Model file for the job. Use its own axes, mm. Face numbers are marked on the shaded views. A direction names the side the tool comes from. Coordinates: 2 decimals unless noted, no trailing zeros. Order: outer loops, then holes, each group sorted by start corner. A loop starts at its lowest first (then second) coordinate and runs counter-clockwise, first axis right, second up.
from build123d import *

# Parameters (mm, degrees)
MODEL_R                 = 1.5
MODEL_W                 = 3
MODEL_H                 = 3
SALIENTE_EXTRUIR1_DEPTH = 3


with BuildPart() as part:
    # Model → Saliente-Extruir1 (new body)
    with BuildSketch(Plane.XY):
        with BuildLine():
            Line((10.993657745, 286.638352596), (10.993657745, 280.893789949))
            ThreePointArc((10.993657745, 280.893789949), (11.107252484, 280.430879899), (11.422229173, 280.073138143))
            ThreePointArc((11.422229173, 280.073138143), (12.115845844, 279.676594232), (12.868657745, 279.408965008))
            ThreePointArc((12.868657745, 279.408965008), (14.499333705, 278.609421111), (15.681157745, 277.230411876))
            ThreePointArc((15.681157745, 277.230411876), (27.493657745, 270.266071273), (39.306157745, 277.230411876))
            ThreePointArc((39.306157745, 277.230411876), (40.487981784, 278.609421111), (42.118657745, 279.408965008))
            ThreePointArc((42.118657745, 279.408965008), (42.871469645, 279.676594232), (43.565086316, 280.073138143))
            ThreePointArc((43.565086316, 280.073138143), (43.880063005, 280.430879899), (43.993657745, 280.893789949))
            Line((43.993657745, 280.893789949), (43.993657745, 286.638352596))
            ThreePointArc((43.993657745, 286.638352596), (43.880063005, 287.101262646), (43.565086316, 287.459004403))
            ThreePointArc((43.565086316, 287.459004403), (42.871469645, 287.855548313), (42.118657745, 288.123177537))
            ThreePointArc((42.118657745, 288.123177537), (40.487981784, 288.922721434), (39.306157745, 290.301730669))
            ThreePointArc((39.306157745, 290.301730669), (27.493657745, 297.266071273), (15.681157745, 290.301730669))
            ThreePointArc((15.681157745, 290.301730669), (14.499333705, 288.922721434), (12.868657745, 288.123177537))
            ThreePointArc((12.868657745, 288.123177537), (12.115845844, 287.855548313), (11.422229173, 287.459004403))
            ThreePointArc((11.422229173, 287.459004403), (11.107252484, 287.101262646), (10.993657745, 286.638352596))
        make_face()
        with Locations((40.993657745, 283.766071273)):
            Circle(MODEL_R, mode=Mode.SUBTRACT)
        with Locations((13.993657745, 283.766071273)):
            Circle(MODEL_R, mode=Mode.SUBTRACT)
        with Locations((27.493657745, 283.766071273)):
            Circle(MODEL_R, mode=Mode.SUBTRACT)
        with Locations((36.493657745, 288.266071273)):
            Rectangle(MODEL_W, MODEL_H, mode=Mode.SUBTRACT)
        with Locations((36.493657745, 279.266071273)):
            Rectangle(MODEL_W, MODEL_H, mode=Mode.SUBTRACT)
        with Locations((18.493657745, 288.266071273)):
            Rectangle(MODEL_W, MODEL_H, mode=Mode.SUBTRACT)
        with Locations((18.493657745, 279.266071273)):
            Rectangle(MODEL_W, MODEL_H, mode=Mode.SUBTRACT)
        with BuildLine():
            Line((30.743657745, 277.391071273), (30.743657745, 279.141071273))
            ThreePointArc((30.743657745, 279.141071273), (30.52398783, 279.671401358), (29.993657745, 279.891071273))
            Line((29.993657745, 279.891071273), (24.993657745, 279.891071273))
            ThreePointArc((24.993657745, 279.891071273), (24.463327659, 279.671401358), (24.243657745, 279.141071273))
            Line((24.243657745, 279.141071273), (24.243657745, 277.391071273))
            ThreePointArc((24.243657745, 277.391071273), (24.463327659, 276.860741187), (24.993657745, 276.641071273))
            Line((24.993657745, 276.641071273), (29.993657745, 276.641071273))
            ThreePointArc((29.993657745, 276.641071273), (30.52398783, 276.860741187), (30.743657745, 277.391071273))
        make_face(mode=Mode.SUBTRACT)
        with BuildLine():
            Line((30.743657745, 290.141071273), (30.743657745, 288.391071273))
            ThreePointArc((30.743657745, 288.391071273), (30.52398783, 287.860741187), (29.993657745, 287.641071273))
            Line((29.993657745, 287.641071273), (24.993657745, 287.641071273))
            ThreePointArc((24.993657745, 287.641071273), (24.463327659, 287.860741187), (24.243657745, 288.391071273))
            Line((24.243657745, 288.391071273), (24.243657745, 290.141071273))
            ThreePointArc((24.243657745, 290.141071273), (24.463327659, 290.671401358), (24.993657745, 290.891071273))
            Line((24.993657745, 290.891071273), (29.993657745, 290.891071273))
            ThreePointArc((29.993657745, 290.891071273), (30.52398783, 290.671401358), (30.743657745, 290.141071273))
        make_face(mode=Mode.SUBTRACT)
    extrude(amount=SALIENTE_EXTRUIR1_DEPTH)


solid = part.part
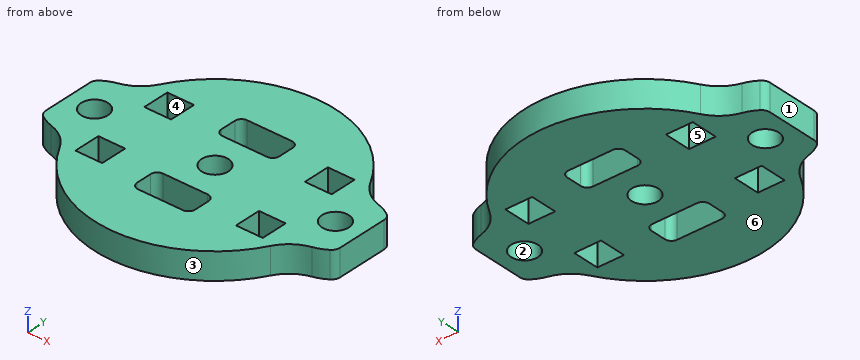
Q1. Cut at D-D, the plane x = 18.5. List the corners of the cut face in (y, z).
Established:
outline: (273.7, 0) - (277.77, 0) - (277.77, 3) - (273.7, 3) - close; (280.77, 0) - (286.77, 0) - (286.77, 3) - (280.77, 3) - close; (289.77, 0) - (293.83, 0) - (293.83, 3) - (289.77, 3) - close
Q2. Probe line 1 (Y direction, x = 27.5, z = 0.95); line 2 (Y direction, x = 36.5, z = 2.75); line 3 (X direction, y = 280, z = 2.65). List the from-to ranges inside material, lowest first.
Established:
line 1: y = 270.27 to 276.64, 279.89 to 282.27, 285.27 to 287.64, 290.89 to 297.27
line 2: y = 273.71 to 277.77, 280.77 to 286.77, 289.77 to 293.82
line 3: x = 11.53 to 16.99, 19.99 to 34.99, 37.99 to 43.46
Q3. Mould opens along Y. For the marked faces 1, 2, 3 and 4 say: pulls with the +Y half, pulls with the -Y half, needs draft (parallel to the pull), parting line crosses it, or undercut.
Established:
face 1: needs draft
face 2: undercut
face 3: pulls with the -Y half
face 4: undercut
Q4. Drop flat-ended pins along their axis: P1, Ø0.9, axis at x = 36, z = 1, coming from the -Y side; P2, Ø1.5, axis at y = 287.5, z = 2, coming from the +X side; P3, Ø1.5, axis at x = 16.5, z = 1.5, coming from the -Y side. Give the stop position or say it passes through.
Established:
P1: stops at y = 272.93
P2: stops at x = 43.99
P3: stops at y = 274.97
Q5. Cut at B-B, the plane x = 26.5. List the corners of the cut face in (y, z), plus the area to 3 significant figures.
Established:
outline: (270.3, 0) - (276.64, 0) - (276.64, 3) - (270.3, 3) - close; (279.89, 0) - (282.64, 0) - (282.64, 3) - (279.89, 3) - close; (284.89, 0) - (287.64, 0) - (287.64, 3) - (284.89, 3) - close; (290.89, 0) - (297.23, 0) - (297.23, 3) - (290.89, 3) - close
area: 54.5 mm2
Q6. Cut at C-C, the plane z = 0.4. Count the separate pieces of the cut face and the enclosed holes in it, plus the area to 3 significant figures.
Established:
separate pieces: 1
enclosed holes: 9
area: 532 mm2
Q7. Which spindle directions (+Z, -Z, +X, -X, +Y, -Y) get a long thin tool onto all of the face, cutting with end or side? Do the marked faces 5 and 6. Say none if no direction does.
Established:
face 5: +Z, -Z
face 6: -Z, +X, -X, +Y, -Y
Q8. Cut at A-A, the plane x = 36. List the corners of the cut face in (y, z).
Established:
outline: (273.28, 0) - (277.77, 0) - (277.77, 3) - (273.28, 3) - close; (280.77, 0) - (286.77, 0) - (286.77, 3) - (280.77, 3) - close; (289.77, 0) - (294.25, 0) - (294.25, 3) - (289.77, 3) - close
